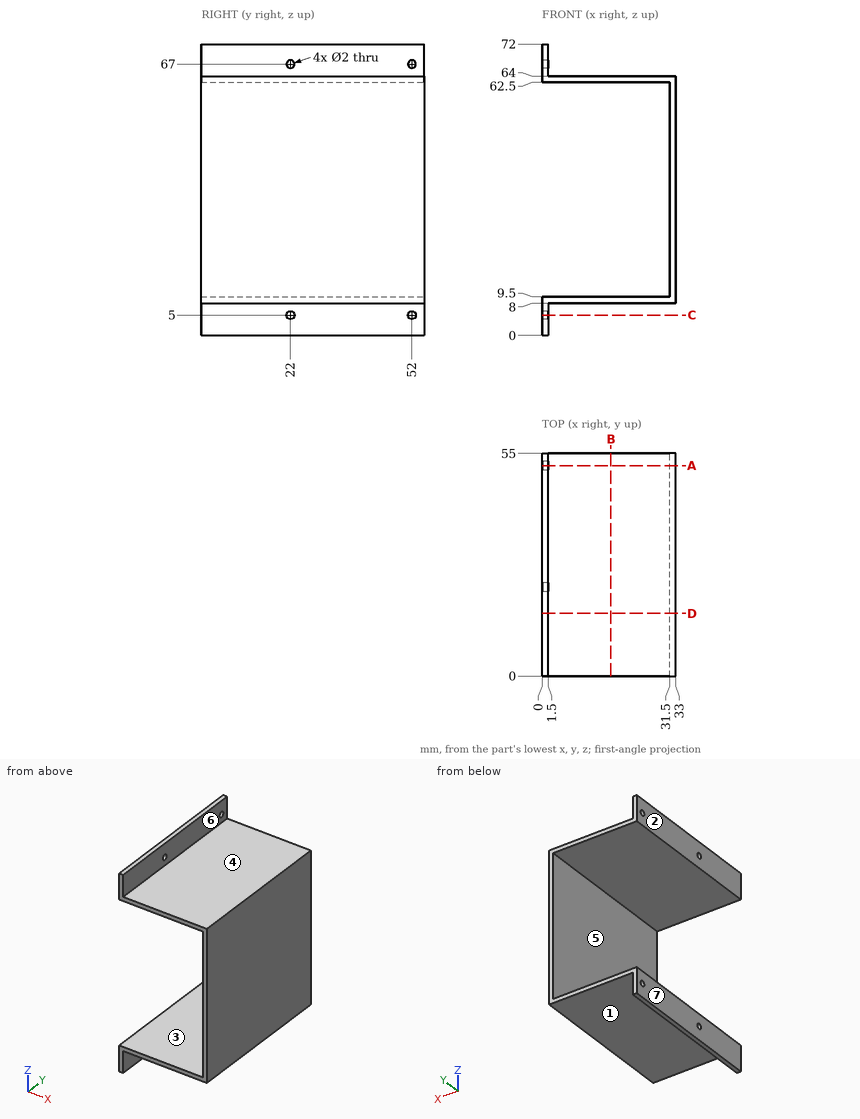
The figure shows three views and two pictorial views of one solid part (mm, origin at its lowest corner). Answer the questions. A direction names the side the tool comes from. Coordinates: 2 decimals unless noted, no trailing zeros. Write each loop counter-clockwise with the first axis right and the second up, starting at its lowest first coordinate (ties: lowest second). Pieces come first, ordered by that corner, then holes. Notation, with made-up numbers: M 68,-10 L 103,-10 A23 ccw 103,4 Z; hole C 19.25,32 d5. An arc over 180 degrees is marked long. Answer as CSV lines item,"result". Start each with the question number.
Item 1: Determine the mould class of the marked faces 1, 2, 3 and 4 for opening direction Z: released by +Z, released by -Z, zero draft, split by the parting line, or undercut.
Item 2: Section B-B on x = 17 is taken. Write down the section's boundary in (y, z), and give its area (3 significant figures).
Item 3: Section C-C on z = 5 is taken. Write down the section's boundary in (x, y).
Item 4: Section A-A on y = 52 is taken. Write down the section's boundary in (x, z), and give its area (4 significant figures).
Item 5: Section D-D on y = 15.5 is taken. Write down the section's boundary in (x, z), and give its area (4 significant figures).
Item 6: A tool of negligible diameter and unlimited length cuts with its end or side. For the marked faces 5, 6 and 7, from which of +Z, -Z, +X, -X, +Y, -Y can it reach the whole face along a straight path? Write none if from no direction.
Item 7: Consider L1, parallel to Z at x = 1.05, y = 22; L2, parallel to Z at x = 26, y = 3.5; L3, parallel to X at y = 30, z = 45. Determine where each line is inside the solid, lowest interval first.
Item 8: Flat-ended cylindrical pins translate along their axes: P1, Ø9, axis at y = 39, z = 69, coming from the +X side; P2, Ø2, axis at x = 19, y = 15.5, coming from the -Z side; P3, Ø3, axis at x = 16, y = 24.5, coming from the +Z side. Find the tip coordinate at first contact, or state that the pin passes through.
Checks:
1,face 1,"released by -Z"
1,face 2,"zero draft"
1,face 3,"undercut"
1,face 4,"released by +Z"
2,outline,"M 0,8 L 55,8 L 55,9.5 L 0,9.5 Z; M 0,62.5 L 55,62.5 L 55,64 L 0,64 Z"
2,area,"165 mm²"
3,outline,"M 0,0 L 1.5,0 L 1.5,21 L 0,21 Z; M 0,23 L 1.5,23 L 1.5,51 L 0,51 Z; M 0,53 L 1.5,53 L 1.5,55 L 0,55 Z"
4,outline,"M 0,0 L 1.5,0 L 1.5,4 L 0,4 Z; M 0,6 L 1.5,6 L 1.5,8 L 33,8 L 33,64 L 1.5,64 L 1.5,66 L 0,66 L 0,62.5 L 31.5,62.5 L 31.5,9.5 L 0,9.5 Z; M 0,68 L 1.5,68 L 1.5,72 L 0,72 Z"
4,area,"196.5 mm²"
5,outline,"M 0,0 L 1.5,0 L 1.5,8 L 33,8 L 33,64 L 1.5,64 L 1.5,72 L 0,72 L 0,62.5 L 31.5,62.5 L 31.5,9.5 L 0,9.5 Z"
5,area,"202.5 mm²"
6,face 5,"-X, +Y, -Y"
6,face 6,"+Z, +X, +Y, -Y"
6,face 7,"+Z, -Z, -X, +Y, -Y"
7,L1,"z = 0 to 4, 6 to 9.5, 62.5 to 66, 68 to 72"
7,L2,"z = 8 to 9.5, 62.5 to 64"
7,L3,"x = 31.5 to 33"
8,P1,"stops at x = 1.5"
8,P2,"stops at z = 8"
8,P3,"stops at z = 64"
